Source: three-view drawing plus pictorial views. Frame: mm from the lowest corner of the part. Coordinates: 2 decimals unless noted, no trailing zeros. Write each loop counter-clockwise with the first axis right and the second up, starting at its lowest first coordinate (ties: lowest second). Pieces come first, ordered by that corner, then holes. Notation, with made-up numbers: M 63,-36.75 L 102,-36.75 A24 ccw 102,-22.75 Z; hole C -13,-26 d4. An arc over 180 degrees is marked long. Write item = value, one per line. Start each with the question number.
Item 1: First-contact query: pin 1 Ø4 at (x, y) = (11.4, 73.6) entering from +Z; pin 2 Ø3 at (x, y) = (73.6, 73.6) entering from +Z. Flat tips, straight axial feed; report the tip coordinate or a pass-through.
Item 2: Section A-A on y = 11.4. Output: boundary loops of the cut face in (x, z), plus the area to 3 significant figures.
Item 3: Ray query, L1, parallel to Y at x = 11.4, z = 1.5; L2, parallel to X at y = 78.5, z = 2.75; L3, parallel to Y at x = 12, z = 2.7. Return the intervals inside material, ascending. Write a range as [from, to].
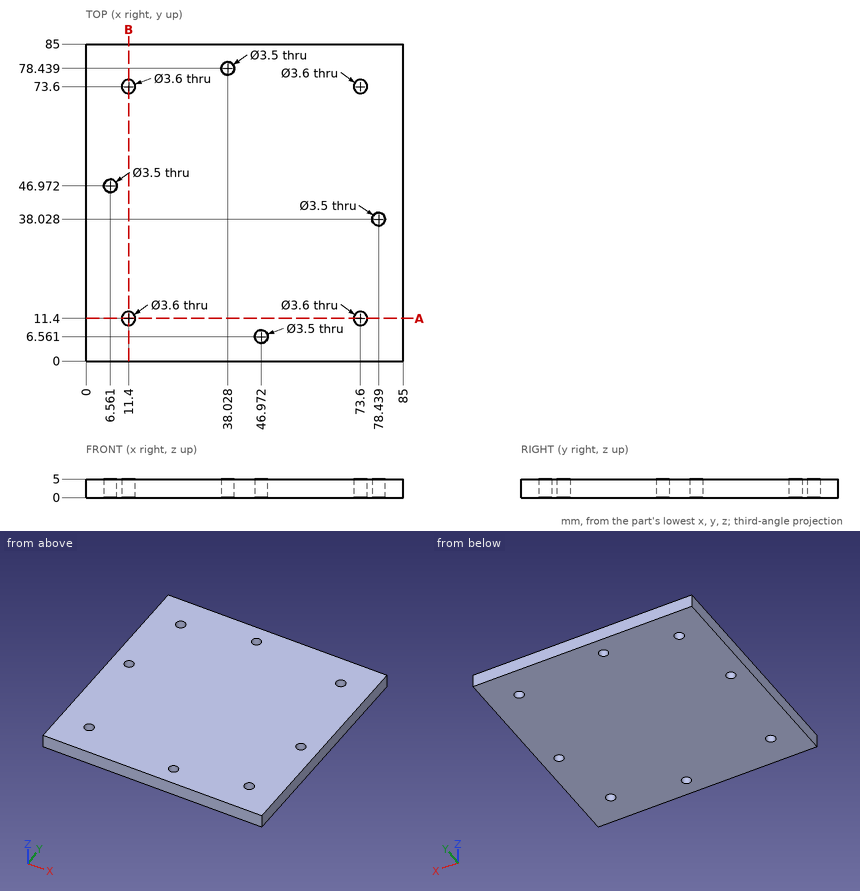
Responses:
q1.pin_1 = 5
q1.pin_2 = through
q2.outline = M 0,0 L 9.6,0 L 9.6,5 L 0,5 Z; M 13.2,0 L 71.8,0 L 71.8,5 L 13.2,5 Z; M 75.4,0 L 85,0 L 85,5 L 75.4,5 Z
q2.area = 389 mm²
q3.L1 = [0, 9.6], [13.2, 71.8], [75.4, 85]
q3.L2 = [0, 36.28], [39.78, 85]
q3.L3 = [0, 9.7], [13.1, 71.9], [75.3, 85]
